Part model, mm, in its own coordinate system. A direction names the side the tool comes from. Give positions to 0.01 mm unless a question says otherwise; leave off trailing zeros. Write each loop counter-clockwise with the first axis right and the second up, starting at its lowest first coordinate (ties: lowest second). Pieces come first, ordered by that corner, then holes. Notation, with made-up numbers: M -30.5,2 L 3.5,2 A25 ccw 3.5,22 Z; hole C 34,24.5 d4. An arc over 180 degrees is marked long. Use a Markdown table: item, result.
```python
from build123d import *

# Parameters (mm, degrees)
F0_W     = 71.63686
F0_H     = 152.34463
F0_R     = 25.373603
F0_W_2   = 22.328374
F0_H_2   = 22.560959
F1_DEPTH = 76.2


with BuildPart() as f1:
    # F0 (on Top) → F1 (new body)
    with BuildSketch(Plane.XY):
        with Locations((0.814056, 0)):
            Rectangle(F0_W, F0_H)
        with Locations((0, -44.307865)):
            Circle(F0_R, mode=Mode.SUBTRACT)
        with Locations((-15.001876, -0.465175)):
            Rectangle(F0_W_2, F0_H_2, mode=Mode.SUBTRACT)
        with Locations((15.001876, -0.465175)):
            Rectangle(F0_W_2, F0_H_2, mode=Mode.SUBTRACT)
        with Locations((0, 44.307865)):
            Circle(F0_R, mode=Mode.SUBTRACT)
    extrude(amount=F1_DEPTH)


solid = f1.part
```
1. Cut at C-C, the plane y = -62. Give the cut face in (x, z).
Findings below:
| item | result |
|---|---|
| outline | M -35,0 L -18.19,0 L -18.19,76.2 L -35,76.2 Z; M 18.19,0 L 36.63,0 L 36.63,76.2 L 18.19,76.2 Z |
2. Cut at B-B, the plane x = -22. Give the cut face in (y, z).
Findings below:
| item | result |
|---|---|
| outline | M -76.17,0 L -56.95,0 L -56.95,76.2 L -76.17,76.2 Z; M -31.67,0 L -11.75,0 L -11.75,76.2 L -31.67,76.2 Z; M 10.82,0 L 31.67,0 L 31.67,76.2 L 10.82,76.2 Z; M 56.95,0 L 76.17,0 L 76.17,76.2 L 56.95,76.2 Z |
3. Drill centre lines: L1, parallel to Y at x = 0, z = 55; L2, parallel to Y at x = -4.5, z = 62.5; L3, parallel to X at y = 44, z = 41.5. Where is each one in solid material? Low to high.
Findings below:
| item | result |
|---|---|
| L1 | -76.17 to -69.68, -18.93 to 18.93, 69.68 to 76.17 |
| L2 | -76.17 to -69.28, -19.34 to -11.75, 10.82 to 19.34, 69.28 to 76.17 |
| L3 | -35 to -25.37, 25.37 to 36.63 |
4. Two-plate mould, pull along X, no slides. Class faces 3 (the flat face through (0, 1, 76.2)), 4 (the flat face through (36.632, -1, 38)), 5 (the cylindrical face through (-5.5, 19.538, 37.567)): released by +X, released by -X, zero draft, split by the parting line, or undercut.
Findings below:
| item | result |
|---|---|
| face 3 | zero draft |
| face 4 | released by +X |
| face 5 | undercut |
5. Cut at A-A, the plane x = 0. Give the cut face in (y, z), then the cut area to 3 significant figures.
Findings below:
| item | result |
|---|---|
| outline | M -76.17,0 L -69.68,0 L -69.68,76.2 L -76.17,76.2 Z; M -18.93,0 L 18.93,0 L 18.93,76.2 L -18.93,76.2 Z; M 69.68,0 L 76.17,0 L 76.17,76.2 L 69.68,76.2 Z |
| area | 3,870 mm2 |
6. Cut at D-D, the plane z = 50. Give the cut face in (x, y).
Findings below:
| item | result |
|---|---|
| outline | M -35,-76.17 L 36.63,-76.17 L 36.63,76.17 L -35,76.17 Z; hole M -26.17,-11.75 L -3.84,-11.75 L -3.84,10.82 L -26.17,10.82 Z; hole C 0,-44.31 d50.75; hole C 0,44.31 d50.75; hole M 3.84,-11.75 L 26.17,-11.75 L 26.17,10.82 L 3.84,10.82 Z |
7. Tool access for faces 1 (the flat face through (-35.004, -1, 38)), 2 (the flat face through (15, 10.815, 38)): list every direction of +Z, -Z, +X, -X, +Y, -Y with a clear straight run to the whole face (end or side of a thin tool).
Findings below:
| item | result |
|---|---|
| face 1 | +Z, -Z, -X, +Y, -Y |
| face 2 | +Z, -Z |
